Study the drawing (mm; zero at the part's minimum x, y, z) and answer. Round coordinates to 2 decimals unless told otherwise and drop trailing zeros. Loops run counter-clockwise (first coordinate to the right, second up) from the corner with the lowest first, then second, coordinate; pieces in that order, holes last. Notation, with made-up numbers: (0.25, 42) -> (6.25, 42) arc R22 cw to (6.25, 49) -> close; hole circle Ø11 at (-9.75, 48). An arc over 180 degrees is marked (long way). Use one line per item in the form item = value.
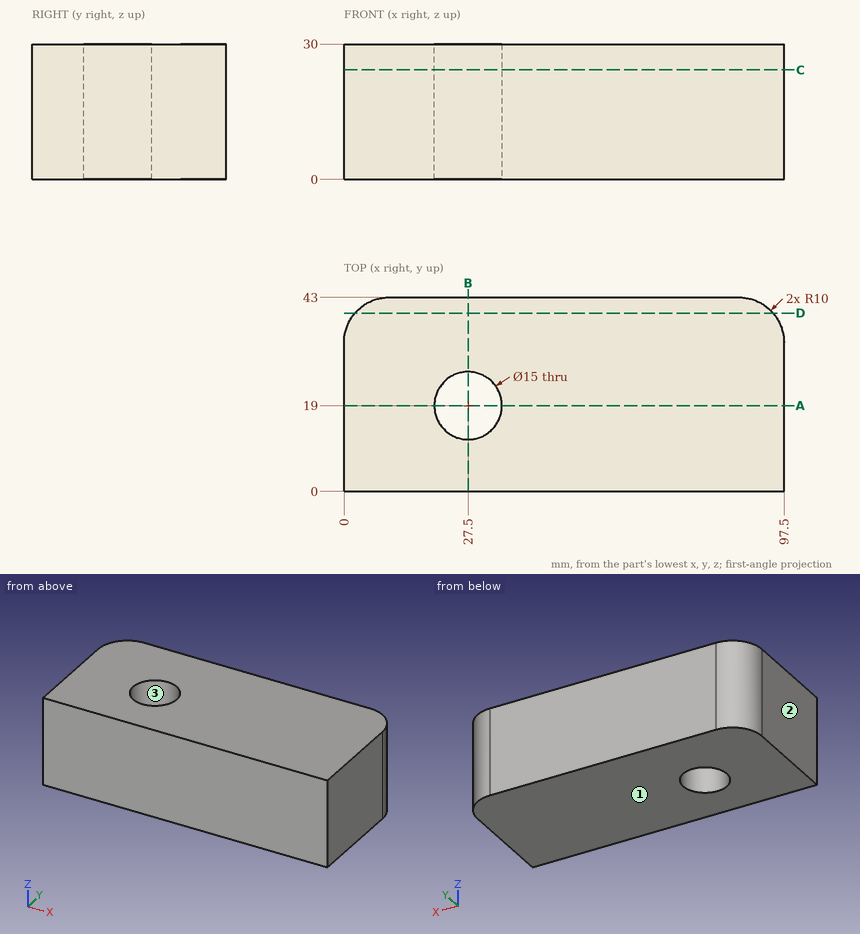
(1) For a pull along X with two mould halves and no side action, classify the marked faces 1, 2 and 3 as +X half, -X half, draft (parallel to the pull), parting line (faces both ways), or undercut.
Completed:
face_1 = draft
face_2 = -X half
face_3 = undercut
(2) Find section C-C, the plane z = 24.25. Write down the section's boundary in (x, y), then the cut area to 3 significant figures.
Completed:
outline = (0, 0) -> (97.5, 0) -> (97.5, 33) arc R10 ccw to (87.5, 43) -> (10, 43) arc R10 ccw to (0, 33) -> close; hole circle Ø15 at (27.5, 19)
area = 3,970 mm2
(3) Consider L1, parallel to Y at x = 27.5, z = 19.25; L2, parallel to X at y = 20, z = 26; L3, parallel to Y at x = 29, z = 27.5. Determine where each line is inside the solid, lowest interval first.
Completed:
L1 = 0 to 11.5, 26.5 to 43
L2 = 0 to 20.07, 34.93 to 97.5
L3 = 0 to 11.65, 26.35 to 43
(4) Find section B-B, the plane x = 27.5. Write down the section's boundary in (y, z), then the cut area to 3 significant figures.
Completed:
outline = (0, 0) -> (11.5, 0) -> (11.5, 30) -> (0, 30) -> close; (26.5, 0) -> (43, 0) -> (43, 30) -> (26.5, 30) -> close
area = 840 mm2
(5) Find section A-A, the plane y = 19. Write down the section's boundary in (x, z).
Completed:
outline = (0, 0) -> (20, 0) -> (20, 30) -> (0, 30) -> close; (35, 0) -> (97.5, 0) -> (97.5, 30) -> (35, 30) -> close
(6) Find section D-D, the plane y = 39.5. Write down the section's boundary in (x, z).
Completed:
outline = (2.4, 0) -> (95.1, 0) -> (95.1, 30) -> (2.4, 30) -> close
